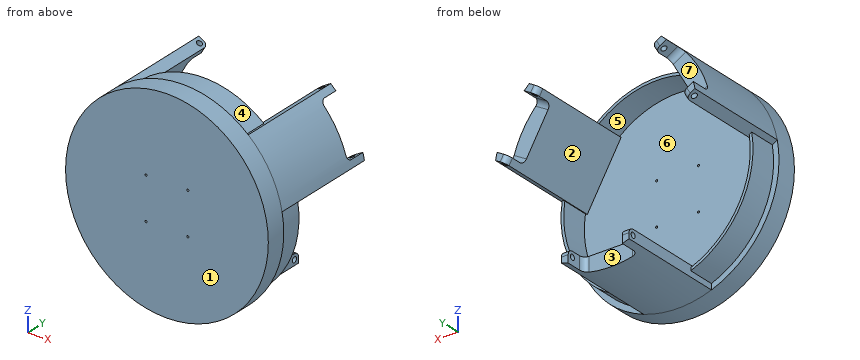
from build123d import *

# Parameters (mm, degrees)
SKETCH1_R                 = 75
BOSS_EXTRUDE1_DEPTH       = 15
BOSS_EXTRUDE2_DEPTH       = 80
CUT_EXTRUDE1_START        = -15
CUT_EXTRUDE1_DEPTH        = 15
F_4_0_MM_DOWEL_HOLES1_D   = 4
FILLET1_R                 = 4
FILLET2_R                 = 4
CIRPATTERN1_COUNT         = 3
FILLET1_OF_CIRPATTERN1_R  = 4
FILLET2_OF_CIRPATTERN1_R  = 4
FORI_ALESATO_1_5MM2_D     = 1.5
SCHIZZO8_R                = 71
SCHIZZO8_R_2              = 69
ESTRUSIONE_SOTTILE1_DEPTH = 20


with BuildPart() as part:
    # Sketch1 → Boss-Extrude1 (new body)
    with BuildSketch(Plane(origin=(0, 0, 0), x_dir=(1, 0, 0), z_dir=(0, 1, 0))):
        with Locations(Location((0, 0, 0), (0, 0, 270))):
            Circle(SKETCH1_R)
    extrude(amount=BOSS_EXTRUDE1_DEPTH)

    # Sketch2 → Boss-Extrude2 (add)
    with BuildSketch(Plane(origin=(0, 15, 0), x_dir=(1, 0, 0), z_dir=(0, 1, 0))):
        with BuildLine():
            Line((-25, 70.710678119), (-25, 62.710678119))
            Line((-25, 62.710678119), (25, 62.710678119))
            Line((25, 62.710678119), (25, 70.710678119))
            ThreePointArc((25, 70.710678119), (0, 75), (-25, 70.710678119))
        make_face()
    boss_extrude2 = extrude(amount=BOSS_EXTRUDE2_DEPTH)

    # Sketch3 → Cut-Extrude1 (cut)
    with BuildSketch(Plane(origin=(0, 95, 0), x_dir=(1, 0, 0), z_dir=(0, 1, 0)).offset(CUT_EXTRUDE1_START)):
        with BuildLine():
            Line((-20, 72.284161474), (-20, 62.710678119))
            Line((-20, 62.710678119), (20, 62.710678119))
            Line((20, 62.710678119), (20, 72.284161474))
            ThreePointArc((20, 72.284161474), (0, 75), (-20, 72.284161474))
        make_face()
    cut_extrude1 = extrude(amount=CUT_EXTRUDE1_DEPTH, mode=Mode.SUBTRACT)

    # Ø4.0 mm Dowel Holes1 (through all)
    with Locations(Plane(origin=(25, 0, 0), x_dir=(0, 0, -1), z_dir=(1, 0, 0))):
        with Locations((66.710678119, 91)):
            f_4_0_mm_dowel_holes1 = Hole(F_4_0_MM_DOWEL_HOLES1_D / 2)

    # Fillet1
    fillet1_edges = [part.edges().sort_by_distance(p)[0] for p in [
        (22.5, 95, -62.710678119),
        (-22.5, 95, -62.710678119),
    ]]
    fillet(fillet1_edges, radius=FILLET1_R)

    # Fillet2
    fillet2_edges = [part.edges().sort_by_distance(p)[0] for p in [
        (20, 80, -67.497419796),
        (-20, 80, -67.497419796),
    ]]
    fillet(fillet2_edges, radius=FILLET2_R)

    # CirPattern1: Boss-Extrude2, Cut-Extrude1, Ø4.0 mm Dowel Holes1 ×3 about axis
    cirpattern1_axis = Axis((0, 0, 0), (0, 1, 0))
    add([boss_extrude2.rotate(cirpattern1_axis, i * 360 / CIRPATTERN1_COUNT) for i in range(1, CIRPATTERN1_COUNT)])
    add([cut_extrude1.rotate(cirpattern1_axis, i * 360 / CIRPATTERN1_COUNT) for i in range(1, CIRPATTERN1_COUNT)], mode=Mode.SUBTRACT)
    add([f_4_0_mm_dowel_holes1.rotate(cirpattern1_axis, i * 360 / CIRPATTERN1_COUNT) for i in range(1, CIRPATTERN1_COUNT)], mode=Mode.SUBTRACT)

    # Fillet1 of CirPattern1
    fillet1_of_cirpattern1_edges = [part.edges().sort_by_distance(p)[0] for p in [
        (-65.559040339, 95, 11.869767474),
        (-43.059040339, 95, 50.840910644),
        (43.059040339, 95, 50.840910644),
        (65.559040339, 95, 11.869767474),
    ]]
    fillet(fillet1_of_cirpattern1_edges, radius=FILLET1_OF_CIRPATTERN1_R)

    # Fillet2 of CirPattern1
    fillet2_of_cirpattern1_edges = [part.edges().sort_by_distance(p)[0] for p in [
        (-68.454480234, 80, 16.428201822),
        (-48.454480234, 80, 51.069217974),
        (48.454480234, 80, 51.069217974),
        (68.454480234, 80, 16.428201822),
    ]]
    fillet(fillet2_of_cirpattern1_edges, radius=FILLET2_OF_CIRPATTERN1_R)

    # Fori Alesato Ø1.5mm2 (through all)
    with Locations(Plane(origin=(0, 0, 0), x_dir=(-1, 0, 0), z_dir=(0, -1, 0))):
        with Locations((-15.499780644, 15.499780644), (15.499780644, -15.499780644), (-15.499780644, -15.499780644), (15.499780644, 15.499780644)):
            Hole(FORI_ALESATO_1_5MM2_D / 2)

    # Schizzo8 → Estrusione-Sottile1 (add)
    with BuildSketch(Plane(origin=(0, 15, 0), x_dir=(1, 0, 0), z_dir=(0, 1, 0))):
        Circle(SCHIZZO8_R)
        Circle(SCHIZZO8_R_2, mode=Mode.SUBTRACT)
    extrude(amount=ESTRUSIONE_SOTTILE1_DEPTH)


solid = part.part
For this review, take the finished solid that the model builds, in its own axes (mm). Face numbers are marked on the shaded views. A direction names the side the tool comes from. Round coordinates to 2 decimals unless told otherwise and drop trailing zeros. Order: outer loops, then holes, each group sorted by start corner. A loop starts at its lowest first (then second) coordinate and runs counter-clockwise, first axis right, second up. Notation, with made-up numbers: (-2.5, -5.75) -> (25.5, -5.75) arc R30 cw to (25.5, 32.25) -> close; hole circle Ø11 at (47, -18). An arc over 180 degrees is marked (long way). Put each result on its own line as item: value.
Q1. For probe 1 along Y at (x, z) = (-16, 16.5); probe 2 along X at (y, z) = (68, 47.5); probe 3 along X at (y, z) = (41, 40.5), list the stretches that pass through material, from the lowest coordinate up. Write a range as [from, to].
Check result:
probe 1: [0, 15]
probe 2: [-58.04, -44.99], [44.99, 58.04]
probe 3: [-63.12, -49.03], [49.03, 63.12]
Q2. Add section A-A on y = 70.5. Write out the cut boundary in (x, z).
Check result:
outline: (-73.74, 13.7) -> (-66.81, 9.7) -> (-41.81, 53.01) -> (-48.74, 57.01) arc R75 ccw to start; (-25, -70.71) arc R75 ccw to (25, -70.71) -> (25, -62.71) -> (-25, -62.71) -> close; (41.81, 53.01) -> (66.81, 9.7) -> (73.74, 13.7) arc R75 ccw to (48.74, 57.01) -> close
Q3. Add section D-D on y = 19. Write out the cut boundary in (x, z), plus the area to 3 significant figures.
Check result:
outline: (-73.74, 13.7) -> (-70.05, 11.58) arc R71 ccw to (-25, -66.45) -> (-25, -70.71) arc R75 ccw to (25, -70.71) -> (25, -66.45) arc R71 ccw to (70.05, 11.58) -> (73.74, 13.7) arc R75 ccw to (48.74, 57.01) -> (45.05, 54.88) arc R71 ccw to (-45.05, 54.88) -> (-48.74, 57.01) arc R75 ccw to start; hole (-68.2, 10.51) arc R69 ccw to (-25, -64.31) -> (-25, -62.71) -> (25, -62.71) -> (25, -64.31) arc R69 ccw to (68.2, 10.51) -> (66.81, 9.7) -> (41.81, 53.01) -> (43.2, 53.81) arc R69 ccw to (-43.2, 53.81) -> (-41.81, 53.01) -> (-66.81, 9.7) -> close
area: 2,200 mm2
Q4. Add section C-C on z = 0. Write out the cut boundary in (x, y), plus the area to 3 significant figures.
Check result:
outline: (-75, 0) -> (75, 0) -> (75, 15) -> (71, 15) -> (71, 35) -> (69, 35) -> (69, 15) -> (-69, 15) -> (-69, 35) -> (-71, 35) -> (-71, 15) -> (-75, 15) -> close
area: 2,330 mm2
Q5. Add section B-B on x = 0. Write out the cut boundary in (y, z).
Check result:
outline: (0, -75) -> (80, -75) -> (80, -62.71) -> (15, -62.71) -> (15, 69) -> (35, 69) -> (35, 71) -> (15, 71) -> (15, 75) -> (0, 75) -> close
Q6. Mouldability with a two-part tool opening along Z and no side actions: class the marked faces 4, 5, 6 and 7 as pulls with the +Z half, pulls with the -Z half, needs draft (parallel to the pull), parting line crosses it, or undercut.
Check result:
face 4: pulls with the +Z half
face 5: undercut
face 6: undercut
face 7: needs draft
Q7. Machinability: for the marked faces 1, 2 and 3, which of the approach directions +Z, -Z, +X, -X, +Y, -Y give a long, thin tool a straight path to every point of the face, cutting with its end or side? Answer none if there is none.
Check result:
face 1: +Z, -Z, +X, -X, -Y
face 2: +Y
face 3: +Z, -Z, +Y
Q8. Insertion check: pin 1 Ø19 at (x, z) = (-20, 63.5) entering from +Y; pin 2 Ø20 at (x, z) = (65, 39.5) entering from +Y; pin 3 Ø10.5 at (y, z) = (88.5, -68) entering from +X; pin 4 Ø10 at (y, z) = (18, 4) entering from -X. Each pin has a flat end and moves straight along its axis. Give the tip position at first contact, or say it passes through.
Check result:
pin 1: y = 35
pin 2: y = 80
pin 3: x = 25
pin 4: x = -75
